Drawing for the job (mm, zero at the part's lowest x, y, z). Give positions to 0.01 mm unless a question says otherwise; leave off trailing zeros. Write each loop counter-clockwise with the first axis right and the second up, starting at its lowest first coordinate (ties: lowest second). Pieces come first, ordered by that corner, then holes. Notation, with made-up numbers: M 14.5,89 L 71.5,89 A12 ccw 71.5,112 Z; hole C -28.5,-21.75 d4. An arc over 180 degrees is marked long. Use a Markdown table: item, result. Add a question column.
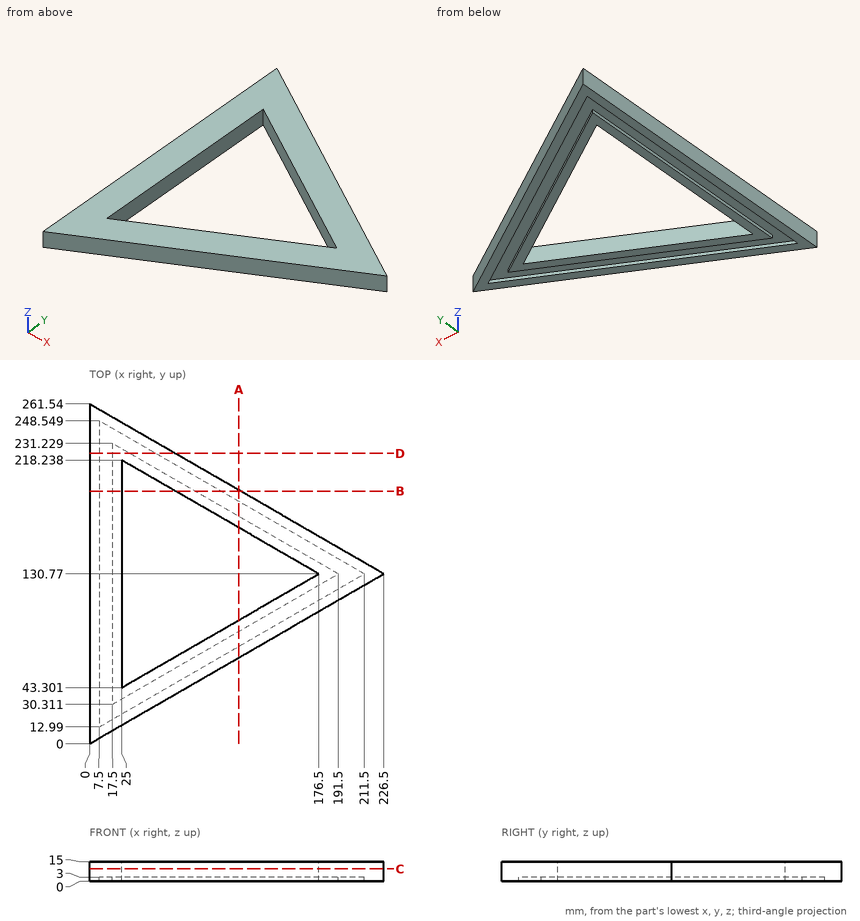
1. Drill centre lines: probe 1 along Y at (x, z) = (70.5, 1.5) (1 decimal); probe 2 along X at (y, z) = (111, 1) (1 decimal); probe 3 along X at (y, z) = (124, 8.25) (1 decimal). Where is each one in solid material? Low to high. Write a range as [from, to].
2. Cut at D-D (y = 223.5). Write the cut outline in (x, z).
3. Cut at B-B (y = 194.5). Write the cut outline in (x, z), then the cut area to 4 significant figures.
4. Flat gauge pins, fed straight in: pin 1 (5 mm diameter, centred on x = 80.5, z = 7.5, fed in from +Y); pin 2 (3 mm diameter, centred on y = 72, z = 5.5, fed in from +X) (1 decimal); pin 3 (3.5 mm diameter, centred on y = 115, z = 2, fed in from +X) (1 decimal). Where does each tip first touch, or does it go through?
5. Cut at A-A (x = 115). Write the cut outline in (y, z) (1 decimal).
6. Cut at C-C (z = 9.5). Write the cut outline in (x, y), then the cut area to 3 significant figures.
A:
| question | item | result |
|---|---|---|
| 1 | probe 1 | y = [40.7, 49.4], [60.9, 69.6], [192, 200.6], [212.2, 220.8] |
| 1 | probe 2 | x = [0, 7.5], [17.5, 25], [142.3, 157.3], [177.3, 192.3] |
| 1 | probe 3 | x = [0, 25], [164.8, 214.8] |
| 2 | outline | M 0,0 L 7.5,0 L 7.5,3 L 17.5,3 L 17.5,0 L 30.89,0 L 30.89,3 L 50.89,3 L 50.89,0 L 65.89,0 L 65.89,15 L 0,15 Z |
| 3 | outline | M 0,0 L 7.5,0 L 7.5,3 L 17.5,3 L 17.5,0 L 25,0 L 25,15 L 0,15 Z; M 66.12,0 L 81.12,0 L 81.12,3 L 101.12,3 L 101.12,0 L 116.12,0 L 116.12,15 L 66.12,15 Z |
| 3 | area | 1,035 mm² |
| 4 | pin 1 | stops at y = 216.51 |
| 4 | pin 2 | stops at x = 127.3 |
| 4 | pin 3 | stops at x = 202.2 |
| 5 | outline | M 66.4,0 L 75.1,0 L 75.1,3 L 86.6,3 L 86.6,0 L 95.3,0 L 95.3,15 L 66.4,15 Z; M 166.3,0 L 174.9,0 L 174.9,3 L 186.5,3 L 186.5,0 L 195.1,0 L 195.1,15 L 166.3,15 Z |
| 6 | outline | M 0,0 L 226.5,130.77 L 0,261.54 Z; hole M 25,43.3 L 176.5,130.77 L 25,218.24 Z |
| 6 | area | 16,400 mm² |
